Read the model definition and answer for the solid it produces. Units are mm, in the model's axes. Face numbers are marked on the shaded views. A direction names the side the tool comes from. Round coordinates to 2 decimals unless told otherwise and drop trailing zeros. Order: outer loops, then holes, each group sorted by start corner. A loop starts at its lowest first (then second) coordinate and runs counter-clockwise, first axis right, second up. Notation, with made-up numbers: (46.25, -24.5) - (102.25, -24.5) arc R30 ccw to (102.25, -1.5) - close; hole circle Ø11 at (49, -5). An arc over 180 degrees is marked (long way). Put each result on its own line as item: value. Start each with the question number.
Q1. For a pull along X with two mould halves and no side action, classify the marked faces 6, 7, 8 and 9 as pulls with the +X half, pulls with the -X half, needs draft (parallel to the pull), parting line crosses it, or undercut.
Q2. Find the intervals of material crossed by line 1 along Y through (x, z) = (74, 7); line 2 along Y through (x, z) = (45, -36); line 3 along Z through (x, y) = (23, 8.5), in increasing order. Write a range as from..to.
Q3. Section C-C on z = -25 is taken. Give the vertices of the cut face in (x, y).
Q4. Each of these flat-tipped pins is pushed along its axis until it touches: pin 1 Ø3 at (x, y) = (54, 28.5) entering from +Z; pin 2 Ø3.5 at (x, z) = (25.5, 19) entering from +Y; pin 3 Ø2.5 at (x, y) = (54, 13.5) entering from -Z; pin 4 Ø8.5 at (x, z) = (74, 19) entering from +Y. Where does it stop, or does it pass through?
Q5. Section D-D on x = 7 is taken. Give the vertices of the cut face in (y, z).
Q6. Section A-A on y = 25.85 is taken. Give the vertices of the cut face in (x, z).
Q7. Which of the six approach directions +Z, -Z, +X, -X, +Y, -Y give full straight-line access (tool end or side, diameter ignored) to the marked faces 1, 2, 3, 4 and 5?
Q8. Section B-B on x = 34.75 is taken. Give the vertices of the cut face in (y, z).
from build123d import *

# Parameters (mm, degrees)
BOSS_EXTRUDE1_DEPTH = 8.75
CUT_EXTRUDE1_DEPTH  = 5
BOSS_EXTRUDE2_DEPTH = 4
BOSS_EXTRUDE3_DEPTH = 4.5
SKETCH5_W           = 84
SKETCH5_H           = 20.25
BOSS_EXTRUDE4_DEPTH = 3.75
BOSS_EXTRUDE5_DEPTH = 4.5
SKETCH7_W           = 40
SKETCH7_H           = 9
SKETCH7_W_2         = 9
SKETCH7_H_2         = 20.25
BOSS_EXTRUDE6_DEPTH = 1
SKETCH8_W           = 40
SKETCH8_H           = 9
BOSS_EXTRUDE7_DEPTH = 1
CHAMFER1_SIZE       = 1
CUT_EXTRUDE2_REACH  = 105.186
SKETCH9_R           = 2.6
CUT_EXTRUDE3_REACH  = 111.522
SKETCH10_R          = 2.6
SKETCH10_W          = 8
SKETCH10_H          = 16
SKETCH12_R          = 4.5
CUT_EXTRUDE4_DEPTH  = 5
CUT_EXTRUDE5_REACH  = 81.494
SKETCH13_R          = 1.6
SKETCH13_R_2        = 13


with BuildPart() as part:
    # Sketch1 → Boss-Extrude1 (new body)
    with BuildSketch(Plane.XY):
        Polygon((0, 0), (84, 0), (84, 47), (15, 47), (0, 32), align=None)
    extrude(amount=BOSS_EXTRUDE1_DEPTH)

    # Sketch2 → Cut-Extrude1 (cut)
    with BuildSketch(Plane(origin=(0, 0, 0), x_dir=(-1, 0, 0), z_dir=(0, 0, -1))):
        Polygon((0, 0), (-44, 0), (-44, 47), (-15, 47), (0, 32), align=None)
    extrude(amount=-CUT_EXTRUDE1_DEPTH, mode=Mode.SUBTRACT)

    # Sketch3 → Boss-Extrude2 (add)
    with BuildSketch(Plane.ZY.offset(-44)):
        Polygon((0, 47), (-38.5, 47), (-42.5, 43), (-42.5, 0), (0, 0), align=None)
    extrude(amount=-BOSS_EXTRUDE2_DEPTH)

    # Sketch4 → Boss-Extrude3 (add)
    with BuildSketch(Plane.XZ):
        Polygon((48, 0), (84, 0), (84, -6.5), (48, -42.5), align=None)
    extrude(amount=-BOSS_EXTRUDE3_DEPTH)

    # Sketch5 → Boss-Extrude4 (add)
    with BuildSketch(Plane.XZ):
        with Locations((42, 18.875)):
            Rectangle(SKETCH5_W, SKETCH5_H)
    extrude(amount=-BOSS_EXTRUDE4_DEPTH)

    # Sketch6 → Boss-Extrude5 (add)
    with BuildSketch(Plane.ZY):
        Polygon((8.75, 3.75), (29, 3.75), (8.75, 24), align=None)
    extrude(amount=-BOSS_EXTRUDE5_DEPTH)

    # Sketch7 → Boss-Extrude6 (add)
    with BuildSketch(Plane(origin=(0, 3.75, 0), x_dir=(1, 0, 0), z_dir=(0, 1, 0))):
        with Locations((64, -19)):
            Rectangle(SKETCH7_W, SKETCH7_H)
        with Locations((14.75, -18.875)):
            Rectangle(SKETCH7_W_2, SKETCH7_H_2)
        with Locations((34.75, -18.875)):
            Rectangle(SKETCH7_W_2, SKETCH7_H_2)
    extrude(amount=BOSS_EXTRUDE6_DEPTH)

    # Sketch8 → Boss-Extrude7 (add)
    with BuildSketch(Plane.XY.offset(8.75)):
        with Locations((64, 14)):
            Rectangle(SKETCH8_W, SKETCH8_H)
        with Locations((64, 34)):
            Rectangle(SKETCH8_W, SKETCH8_H)
    extrude(amount=BOSS_EXTRUDE7_DEPTH)

    # Chamfer1
    chamfer1_edges = [part.edges().sort_by_distance(p)[0] for p in [
        (19.25, 4.75, 18.875),
        (14.75, 4.75, 29),
        (10.25, 4.75, 18.875),
        (30.25, 4.75, 18.875),
        (34.75, 4.75, 29),
        (39.25, 4.75, 18.875),
        (64, 4.75, 14.5),
        (64, 4.75, 23.5),
        (44, 4.75, 19),
        (64, 29.5, 9.75),
        (44, 34, 9.75),
        (64, 38.5, 9.75),
        (64, 9.5, 9.75),
        (64, 18.5, 9.75),
        (44, 14, 9.75),
    ]]
    chamfer(chamfer1_edges, length=CHAMFER1_SIZE - 0.0001)  # a hair under: the kernel refuses the full size

    # Sketch9 → Cut-Extrude2 (cut, up to next)
    with BuildSketch(Plane(origin=(0, 4.75, 0), x_dir=(1, 0, 0), z_dir=(0, 1, 0)), mode=Mode.PRIVATE) as cut_extrude2_sk1:
        with Locations(Location((14.75, -19, 0), (0, 0, 180))):
            Circle(SKETCH9_R)
    cut_extrude2_tool1 = extrude(cut_extrude2_sk1.sketch, amount=-CUT_EXTRUDE2_REACH, mode=Mode.PRIVATE) & part.part
    # Sketch9 → Cut-Extrude2 (cut, up to next)
    with BuildSketch(Plane(origin=(0, 4.75, 0), x_dir=(1, 0, 0), z_dir=(0, 1, 0)), mode=Mode.PRIVATE) as cut_extrude2_sk2:
        with Locations(Location((34.75, -19, 0), (0, 0, 180))):
            Circle(SKETCH9_R)
    cut_extrude2_tool2 = extrude(cut_extrude2_sk2.sketch, amount=-CUT_EXTRUDE2_REACH, mode=Mode.PRIVATE) & part.part
    # Sketch9 → Cut-Extrude2 (cut, up to next)
    with BuildSketch(Plane(origin=(0, 4.75, 0), x_dir=(1, 0, 0), z_dir=(0, 1, 0)), mode=Mode.PRIVATE) as cut_extrude2_sk3:
        with Locations(Location((54, -19, 0), (0, 0, 180))):
            Circle(SKETCH9_R)
    cut_extrude2_tool3 = extrude(cut_extrude2_sk3.sketch, amount=-CUT_EXTRUDE2_REACH, mode=Mode.PRIVATE) & part.part
    # Sketch9 → Cut-Extrude2 (cut, up to next)
    with BuildSketch(Plane(origin=(0, 4.75, 0), x_dir=(1, 0, 0), z_dir=(0, 1, 0)), mode=Mode.PRIVATE) as cut_extrude2_sk4:
        with Locations(Location((74, -19, 0), (0, 0, 180))):
            Circle(SKETCH9_R)
    cut_extrude2_tool4 = extrude(cut_extrude2_sk4.sketch, amount=-CUT_EXTRUDE2_REACH, mode=Mode.PRIVATE) & part.part
    add(cut_extrude2_tool1.solids().sort_by_distance((14.75, 4.75, 19))[0], mode=Mode.SUBTRACT)
    add(cut_extrude2_tool2.solids().sort_by_distance((34.75, 4.75, 19))[0], mode=Mode.SUBTRACT)
    add(cut_extrude2_tool3.solids().sort_by_distance((54, 4.75, 19))[0], mode=Mode.SUBTRACT)
    add(cut_extrude2_tool4.solids().sort_by_distance((74, 4.75, 19))[0], mode=Mode.SUBTRACT)

    # Sketch10 → Cut-Extrude3 (cut, up to next)
    with BuildSketch(Plane.XY.offset(9.75), mode=Mode.PRIVATE) as cut_extrude3_sk1:
        with Locations((54, 34)):
            Circle(SKETCH10_R)
    cut_extrude3_tool1 = extrude(cut_extrude3_sk1.sketch, amount=-CUT_EXTRUDE3_REACH, mode=Mode.PRIVATE) & part.part
    # Sketch10 → Cut-Extrude3 (cut, up to next)
    with BuildSketch(Plane.XY.offset(9.75), mode=Mode.PRIVATE) as cut_extrude3_sk2:
        with Locations((74, 34)):
            Circle(SKETCH10_R)
    cut_extrude3_tool2 = extrude(cut_extrude3_sk2.sketch, amount=-CUT_EXTRUDE3_REACH, mode=Mode.PRIVATE) & part.part
    # Sketch10 → Cut-Extrude3 (cut, up to next)
    with BuildSketch(Plane.XY.offset(9.75), mode=Mode.PRIVATE) as cut_extrude3_sk3:
        with Locations((54, 14)):
            Circle(SKETCH10_R)
    cut_extrude3_tool3 = extrude(cut_extrude3_sk3.sketch, amount=-CUT_EXTRUDE3_REACH, mode=Mode.PRIVATE) & part.part
    # Sketch10 → Cut-Extrude3 (cut, up to next)
    with BuildSketch(Plane.XY.offset(9.75), mode=Mode.PRIVATE) as cut_extrude3_sk4:
        with Locations((74, 14)):
            Circle(SKETCH10_R)
    cut_extrude3_tool4 = extrude(cut_extrude3_sk4.sketch, amount=-CUT_EXTRUDE3_REACH, mode=Mode.PRIVATE) & part.part
    # Sketch10 → Cut-Extrude3 (cut, up to next)
    with BuildSketch(Plane.XY.offset(9.75), mode=Mode.PRIVATE) as cut_extrude3_sk5:
        with Locations((34.75, 14)):
            Circle(SKETCH10_R)
    cut_extrude3_tool5 = extrude(cut_extrude3_sk5.sketch, amount=-CUT_EXTRUDE3_REACH, mode=Mode.PRIVATE) & part.part
    # Sketch10 → Cut-Extrude3 (cut, up to next)
    with BuildSketch(Plane.XY.offset(9.75), mode=Mode.PRIVATE) as cut_extrude3_sk6:
        with Locations((14.75, 14)):
            Circle(SKETCH10_R)
    cut_extrude3_tool6 = extrude(cut_extrude3_sk6.sketch, amount=-CUT_EXTRUDE3_REACH, mode=Mode.PRIVATE) & part.part
    # Sketch10 → Cut-Extrude3 (cut, up to next)
    with BuildSketch(Plane.XY.offset(9.75), mode=Mode.PRIVATE) as cut_extrude3_sk7:
        with Locations((34.75, 27)):
            Rectangle(SKETCH10_W, SKETCH10_H)
    cut_extrude3_tool7 = extrude(cut_extrude3_sk7.sketch, amount=-CUT_EXTRUDE3_REACH, mode=Mode.PRIVATE) & part.part
    add(cut_extrude3_tool1.solids().sort_by_distance((54, 34, 9.75))[0], mode=Mode.SUBTRACT)
    add(cut_extrude3_tool2.solids().sort_by_distance((74, 34, 9.75))[0], mode=Mode.SUBTRACT)
    add(cut_extrude3_tool3.solids().sort_by_distance((54, 14, 9.75))[0], mode=Mode.SUBTRACT)
    add(cut_extrude3_tool4.solids().sort_by_distance((74, 14, 9.75))[0], mode=Mode.SUBTRACT)
    add(cut_extrude3_tool5.solids().sort_by_distance((34.75, 14, 9.75))[0], mode=Mode.SUBTRACT)
    add(cut_extrude3_tool6.solids().sort_by_distance((14.75, 14, 9.75))[0], mode=Mode.SUBTRACT)
    add(cut_extrude3_tool7.solids().sort_by_distance((34.75, 27, 9.75))[0], mode=Mode.SUBTRACT)

    # Sketch12 → Cut-Extrude4 (cut)
    with BuildSketch(Plane(origin=(0, 0, 0), x_dir=(-1, 0, 0), z_dir=(0, 0, -1))):
        with Locations((-54, 34)):
            Circle(SKETCH12_R)
        with Locations((-74, 34)):
            Circle(SKETCH12_R)
        with Locations((-74, 14)):
            Circle(SKETCH12_R)
        with Locations((-54, 14)):
            Circle(SKETCH12_R)
    extrude(amount=-CUT_EXTRUDE4_DEPTH, mode=Mode.SUBTRACT)

    # Sketch13 → Cut-Extrude5 (cut, up to next)
    with BuildSketch(Plane(origin=(48, 0, 0), x_dir=(0, 0, -1), z_dir=(1, 0, 0)), mode=Mode.PRIVATE) as cut_extrude5_sk1:
        with Locations((5.85, 41.35)):
            Circle(SKETCH13_R)
    cut_extrude5_tool1 = extrude(cut_extrude5_sk1.sketch, amount=-CUT_EXTRUDE5_REACH, mode=Mode.PRIVATE) & part.part
    # Sketch13 → Cut-Extrude5 (cut, up to next)
    with BuildSketch(Plane(origin=(48, 0, 0), x_dir=(0, 0, -1), z_dir=(1, 0, 0)), mode=Mode.PRIVATE) as cut_extrude5_sk2:
        with Locations((36.85, 41.35)):
            Circle(SKETCH13_R)
    cut_extrude5_tool2 = extrude(cut_extrude5_sk2.sketch, amount=-CUT_EXTRUDE5_REACH, mode=Mode.PRIVATE) & part.part
    # Sketch13 → Cut-Extrude5 (cut, up to next)
    with BuildSketch(Plane(origin=(48, 0, 0), x_dir=(0, 0, -1), z_dir=(1, 0, 0)), mode=Mode.PRIVATE) as cut_extrude5_sk3:
        with Locations((36.85, 10.5)):
            Circle(SKETCH13_R)
    cut_extrude5_tool3 = extrude(cut_extrude5_sk3.sketch, amount=-CUT_EXTRUDE5_REACH, mode=Mode.PRIVATE) & part.part
    # Sketch13 → Cut-Extrude5 (cut, up to next)
    with BuildSketch(Plane(origin=(48, 0, 0), x_dir=(0, 0, -1), z_dir=(1, 0, 0)), mode=Mode.PRIVATE) as cut_extrude5_sk4:
        with Locations((5.85, 10.5)):
            Circle(SKETCH13_R)
    cut_extrude5_tool4 = extrude(cut_extrude5_sk4.sketch, amount=-CUT_EXTRUDE5_REACH, mode=Mode.PRIVATE) & part.part
    # Sketch13 → Cut-Extrude5 (cut, up to next)
    with BuildSketch(Plane(origin=(48, 0, 0), x_dir=(0, 0, -1), z_dir=(1, 0, 0)), mode=Mode.PRIVATE) as cut_extrude5_sk5:
        with Locations((21.35, 25.85)):
            Circle(SKETCH13_R_2)
    cut_extrude5_tool5 = extrude(cut_extrude5_sk5.sketch, amount=-CUT_EXTRUDE5_REACH, mode=Mode.PRIVATE) & part.part
    add(cut_extrude5_tool1.solids().sort_by_distance((48, 41.35, -5.85))[0], mode=Mode.SUBTRACT)
    add(cut_extrude5_tool2.solids().sort_by_distance((48, 41.35, -36.85))[0], mode=Mode.SUBTRACT)
    add(cut_extrude5_tool3.solids().sort_by_distance((48, 10.5, -36.85))[0], mode=Mode.SUBTRACT)
    add(cut_extrude5_tool4.solids().sort_by_distance((48, 10.5, -5.85))[0], mode=Mode.SUBTRACT)
    add(cut_extrude5_tool5.solids().sort_by_distance((48, 25.85, -21.35))[0], mode=Mode.SUBTRACT)


solid = part.part
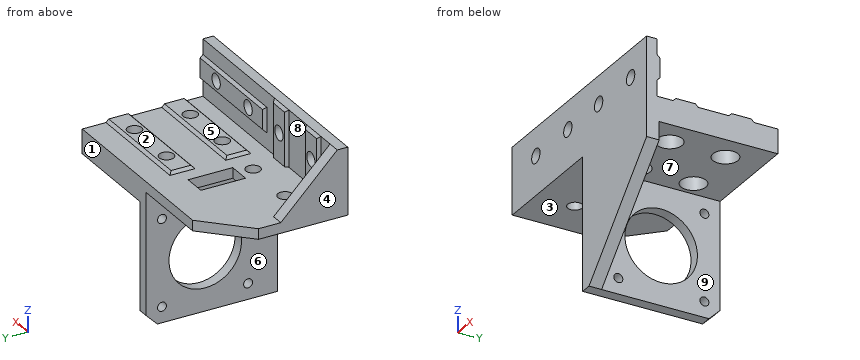
Findings:
1. face 6: pulls with the -X half
1. face 7: needs draft
1. face 8: undercut
1. face 9: pulls with the +X half
2. line 1: 0..11.4, 16.6..31.4, 36.6..47
2. line 2: 0..9.14, 11.86..39.99, 42.71..47
2. line 3: 5..8.75
3. outline: (44, 0) - (65.5, 0) - (65.5, 4.5) - (48, 4.5) - (48, 13.37) - (44, 13.37) - close; (44, 38.33) - (48, 38.33) - (48, 47) - (44, 47) - close
4. pin 1: z = 9.25
4. pin 2: y = 3.75
4. pin 3: through
4. pin 4: y = 4.75
5. outline: (0, 5) - (39, 5) - (39, 8.75) - (3.75, 8.75) - (3.75, 29) - (0, 29) - close
6. outline: (0, 5) - (30.75, 5) - (30.75, 8.75) - (0, 8.75) - close; (38.75, 5) - (44, 5) - (44, -8.35) - (48, -8.35) - (48, 0) - (84, 0) - (84, 8.75) - (38.75, 8.75) - close; (44, -42.5) - (48, -42.5) - (48, -34.35) - (44, -34.35) - close
7. face 1: +Z, -Z, +X, -X, +Y
7. face 2: +Z, +X, -X, +Y
7. face 3: -Z, -X, +Y, -Y
7. face 4: +Z, -Z, -X, +Y, -Y
7. face 5: +Z, +X, +Y
8. outline: (0, 5) - (11.4, 5) - (11.4, 8.75) - (4.75, 8.75) - (4.75, 16.4) - (0, 16.4) - close; (0, 21.6) - (4.75, 21.6) - (4.75, 28) - (3.75, 29) - (0, 29) - close; (16.6, 5) - (19, 5) - (19, 8.75) - (16.6, 8.75) - close; (35, 5) - (47, 5) - (47, 8.75) - (35, 8.75) - close
